Could you check a few things on this model? Use its own coordinates, in mm. Face numbers are marked on the shaded views. Coordinates: 2 decimals unless noted, no trailing zeros. Loops run counter-clockwise (first coordinate to the right, second up) from the corner with the lowest first, then second, coordinate; pieces in that order, holes last.
1) Imagine slicing it at A-A on x = 12.5. Please give me the cut outline in (y, z).
2) If I drill on line 1 along X through (y, z) = (16, 4); line 2 along Y through (x, z) = (-8.5, 0.5); line 3 along Z through (x, y) = (1, 11), over which ranges is the centre line in solid material (lowest first)?
3) Thinking about a two-plate mould opening in Y: for the marked faces 1, 2 and 3, which applies, released by +Y, released by -Y, zero draft, split by the parting line, or undercut?
4) Imagine slicing it at D-D on y = -11. Please give me the cut outline in (x, z), plus the area to 3 significant figures.
5) Imagine slicing it at B-B on z = 3. Please give me the cut outline in (x, y), plus the area to 3 significant figures.
6) Will these pins go through, and if not, where does the flat tip stop? P1, Ø1.1, axis at y = 12.5, z = 2.5, coming from the -X side; P2, Ø2, axis at x = -12, y = 32, coming from the +Z side; P3, Ø5, axis at x = 49, y = -17.5, coming from the +Z side.
7) Imagine slicing it at C-C on y = 26. Please give me the cut outline in (x, z), plus the area to 3 significant figures.
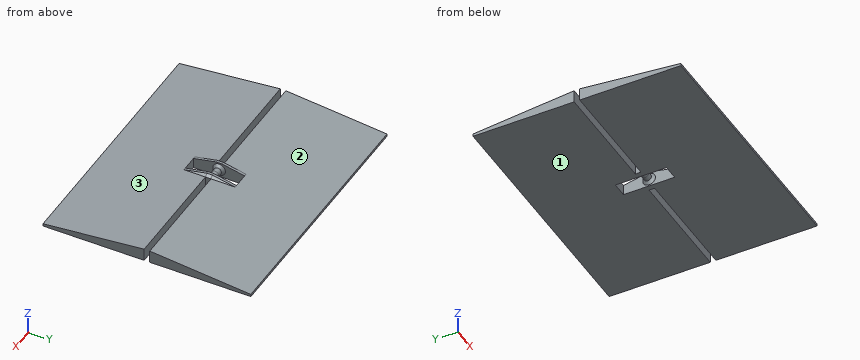
```python
from build123d import *

# Parameters (mm, degrees)
DODANIE_WYCI_GNI_CIE1_DEPTH = 1
DODANIE_WYCI_GNI_CIE2_DEPTH = 100
SZKIC3_W                    = 6
SZKIC3_H                    = 9
WYTNIJ_WYCI_GNI_CIE1_DEPTH  = 10
SZKIC4_W                    = 2
SZKIC4_H                    = 5
DODANIE_WYCI_GNI_CIE3_DEPTH = 1.1
DODANIE_WYCI_GNI_CIE5_DEPTH = 2
SZKIC8_R                    = 2.5
SZKIC9_R                    = 1.45
SZKIC10_R                   = 1.45
DODANIE_WYCI_GNI_CIE6_DEPTH = 2
SFAZOWANIE1_SIZE            = 1


with BuildPart() as part:
    # Szkic1 → Dodanie-wyciągnięcie1 (new body)
    with BuildSketch(Plane.XY):
        Polygon((15.316574048, 11.214895549), (-29.683425952, 11.214895549), (-29.683425952, -28.685104451), (70.316574048, -28.685104451), (70.316574048, 11.214895549), (25.316574048, 11.214895549), align=None)
    extrude(amount=DODANIE_WYCI_GNI_CIE1_DEPTH)

    # Szkic2 → Dodanie-wyciągnięcie2 (add)
    with BuildSketch(Plane.ZY.offset(29.683425952)):
        Polygon((1, 11.214895549), (5, 11.214895549), (1, -28.685104451), align=None)
    extrude(amount=-DODANIE_WYCI_GNI_CIE2_DEPTH)

    # Szkic3 → Wytnij-wyciągnięcie1 (cut)
    with BuildSketch(Plane(origin=(0, 0, 0), x_dir=(-1, 0, 0), z_dir=(0, 0, -1))):
        with Locations((-20.316574048, 6.714895549)):
            Rectangle(SZKIC3_W, SZKIC3_H)
    extrude(amount=-WYTNIJ_WYCI_GNI_CIE1_DEPTH, mode=Mode.SUBTRACT)

    # Szkic4 → Dodanie-wyciągnięcie3 (add)
    with BuildSketch(Plane(origin=(0, 11.214895549, 0), x_dir=(1, 0, 0), z_dir=(0, 1, 0))):
        with Locations((24.316574048, -2.5)):
            Rectangle(SZKIC4_W, SZKIC4_H)
        with Locations((16.316574048, -2.5)):
            Rectangle(SZKIC4_W, SZKIC4_H)
    extrude(amount=DODANIE_WYCI_GNI_CIE3_DEPTH)

    # Lustro2: part across plane


with BuildPart() as part_1:
    add(part.part)
    add(part.part.mirror(Plane.ZX.offset(12.314895549)))

    # Szkic7 → Dodanie-wyciągnięcie5 (add)
    with BuildSketch(Plane.ZY.offset(-23.316574048)):
        Polygon((4.097744361, 22.414895549), (5, 13.414895549), (5, 11.214895549), (4.097744361, 2.214895549), (6, 11.214895549), (6, 13.414895549), align=None)
    dodanie_wyci_gni_cie5 = extrude(amount=-DODANIE_WYCI_GNI_CIE5_DEPTH)

    # Szkic8 → Wyciągnięcie po profilach1 section 0
    with BuildSketch(Plane.ZY.offset(-23.316574048)):
        with Locations((3, 12.314895549)):
            Circle(SZKIC8_R)
    # Szkic9 → Wyciągnięcie po profilach1 section 1
    with BuildSketch(Plane.ZY.offset(-22.316574048)):
        with Locations((3, 12.314895549)):
            Circle(SZKIC9_R)
    wyci_gni_cie_po_profilach1 = loft()

    # Szkic10 → Dodanie-wyciągnięcie6 (add)
    with BuildSketch(Plane.ZY.offset(-22.316574048)):
        with Locations((3, 12.314895549)):
            Circle(SZKIC10_R)
    dodanie_wyci_gni_cie6 = extrude(amount=DODANIE_WYCI_GNI_CIE6_DEPTH)

    # Lustro3: Dodanie-wyciągnięcie5, Wyciągnięcie po profilach1, Dodanie-wyciągnięcie6 across plane
    add(dodanie_wyci_gni_cie5.mirror(Plane(origin=(20.316574048, 12.314895549, 3), x_dir=(0, 0, 1), z_dir=(-1, 0, 0))))
    add(wyci_gni_cie_po_profilach1.mirror(Plane(origin=(20.316574048, 12.314895549, 3), x_dir=(0, 0, 1), z_dir=(-1, 0, 0))))
    add(dodanie_wyci_gni_cie6.mirror(Plane(origin=(20.316574048, 12.314895549, 3), x_dir=(0, 0, 1), z_dir=(-1, 0, 0))))

    # Sfazowanie1
    sfazowanie1_edges = [part_1.edges().sort_by_distance(p)[0] for p in [
        (15.316574048, 6.714895549, 5.04887218),
        (15.316574048, 12.314895549, 6),
        (15.316574048, 17.914895549, 5.04887218),
        (25.316574048, 17.914895549, 5.04887218),
        (25.316574048, 12.314895549, 6),
        (25.316574048, 6.714895549, 5.04887218),
    ]]
    chamfer(sfazowanie1_edges, length=SFAZOWANIE1_SIZE)


solid = part_1.part
```
Filled in:
1. outline: (-28.69, 0) - (11.21, 0) - (11.21, 5) - (-28.69, 1) - close; (13.41, 0) - (53.31, 0) - (53.31, 1) - (13.41, 5) - close
2. line 1: x = -29.68 to 17.32, 23.32 to 70.32
2. line 2: y = -28.69 to 11.21, 13.41 to 53.31
2. line 3: z = 0 to 4.98
3. face 1: zero draft
3. face 2: released by +Y
3. face 3: released by -Y
4. outline: (-29.68, 0) - (70.32, 0) - (70.32, 2.77) - (-29.68, 2.77) - close
4. area: 277 mm2
5. outline: (-29.68, -8.74) - (70.32, -8.74) - (70.32, 11.21) - (25.32, 11.21) - (25.32, 13.41) - (70.32, 13.41) - (70.32, 33.36) - (-29.68, 33.36) - (-29.68, 13.41) - (15.32, 13.41) - (15.32, 11.21) - (-29.68, 11.21) - close; hole (17.32, 2.21) - (23.32, 2.21) - (23.32, 9.81) - (22.32, 10.86) - (18.32, 10.86) - (17.32, 9.81) - close; hole (17.32, 14.81) - (18.32, 13.76) - (22.32, 13.76) - (23.32, 14.81) - (23.32, 22.41) - (17.32, 22.41) - close
5. area: 3,910 mm2
6. P1: stops at x = 15.32
6. P2: stops at z = 3.24
6. P3: stops at z = 2.37
7. outline: (-29.68, 0) - (70.32, 0) - (70.32, 3.74) - (-29.68, 3.74) - close
7. area: 374 mm2
